from build123d import *

# Parameters (mm, degrees)
F0_W    = 20
F0_H    = 49
F3_D    = 16.5
F4_SIZE = 1.5


with BuildPart() as f1:
    # F0 (on Front) → F1 (revolve)
    with BuildSketch(Plane.XZ):
        with Locations((10, 24.5)):
            Rectangle(F0_W, F0_H)
    revolve(axis=Axis((0, 0, 21.905942), (0, 0, 1)))

    # F3 (through all)
    with Locations(Plane.XY.offset(49)):
        with Locations((0, 0)):
            Hole(F3_D / 2)

    # F4
    f4_edges = [f1.edges().sort_by_distance(p)[0] for p in [
        (-20, 0, 49),
        (-20, 0, 0),
    ]]
    chamfer(f4_edges, length=F4_SIZE)


solid = f1.part
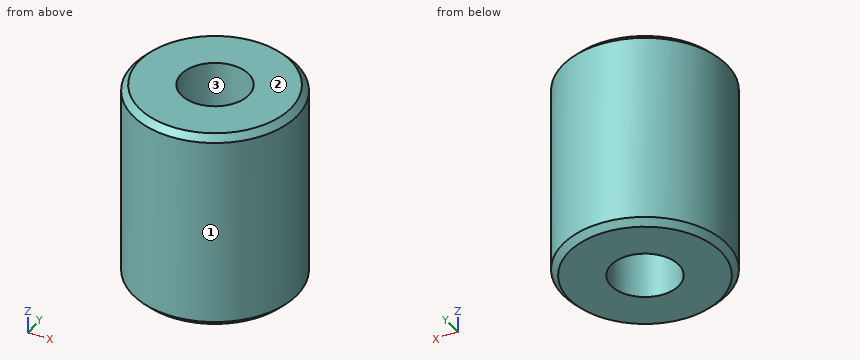
Build history of the part. All positions in model axes, mm. Face numbers are marked on the shaded views. Round coordinates to 2 decimals unless told otherwise and drop trailing zeros. Loops run counter-clockwise (first coordinate to the right, second up) from the corner with the lowest first, then second, coordinate; pieces in that order, holes last. Notation, with made-up numbers: (-21, -37) -> (24, -37) arc R30 cw to (24, -9) -> close; hole circle Ø11 at (68, -35.5). An arc over 180 degrees is marked (long way). One line per item, written item: value. Start each with the question number.
Q1. Probe line 1 along Y through (x, z) = (0, 11.5); line 2 along X through (y, z) = (-3.5, 14); line 3 along X through (y, z) = (10, 35). List the from-to ranges inside material, lowest first.
Q2. Drop flat-ended pins along their axis: pin 1 Ø13 at (x, y) = (0, 0) entering from +Z; pin 2 Ø1.5 at (x, y) = (-16, -11) entering from -Z; pin 3 Ø2 at (y, z) = (-4, 36.5) entering from +X; pin 4 Ø2 at (x, z) = (8, 23) entering from -Y (3 decimals). Give the stop position or say it passes through.
Q3. Two-plate mould, pull along X, no slides. Class the marked faces 1, 2 and 3: released by +X, released by -X, zero draft, split by the parting line, or undercut.
Q4. Cut at C-C on z = 36. List the corners of the cut face in (x, y).
Q5. Cut at A-A on y = 0. List the corners of the cut face in (x, z), plus the area to 3 significant figures.
Computed:
1. line 1: -20 to -8.25, 8.25 to 20
1. line 2: -19.69 to -7.47, 7.47 to 19.69
1. line 3: -17.32 to 17.32
2. pin 1: through
2. pin 2: z = 0.17
2. pin 3: x = 19.77
2. pin 4: y = -18.735
3. face 1: split by the parting line
3. face 2: zero draft
3. face 3: undercut
4. outline: circle Ø40 at (0, 0); hole circle Ø16.5 at (0, 0)
5. outline: (-20, 1.5) -> (-18.5, 0) -> (-8.25, 0) -> (-8.25, 49) -> (-18.5, 49) -> (-20, 47.5) -> close; (8.25, 0) -> (18.5, 0) -> (20, 1.5) -> (20, 47.5) -> (18.5, 49) -> (8.25, 49) -> close
5. area: 1,150 mm²
